Read the model definition and answer for the solid it produces. Units are mm, in the model's axes. Give positions to 0.01 mm unless a question says otherwise; leave off trailing zeros. Loops run counter-clockwise (first coordinate to the right, second up) from the corner with the lowest first, then second, coordinate; pieces in that order, holes last. Notation, with made-up numbers: (-12, 18.25) - (11, 18.25) arc R24 ccw to (11, 54.25) - close; hole circle Ø11 at (-31, 52.5). An arc over 180 degrees is marked (long way). Write item = value, one per line.
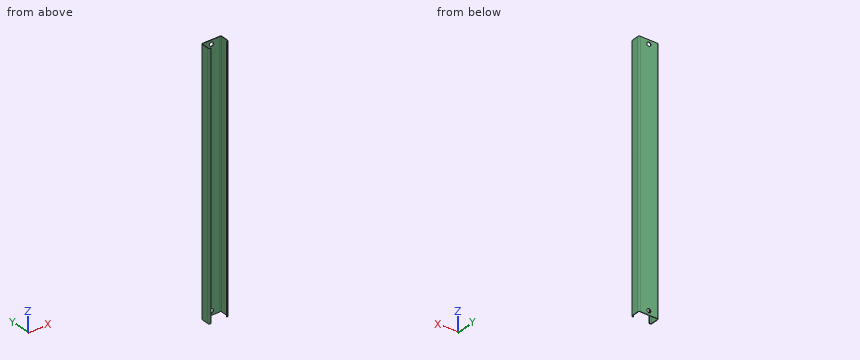
```python
from build123d import *

# Parameters (mm, degrees)
PAD001_DEPTH    = 572
SKETCH004_R     = 4.5
POCKET002_DEPTH = 5
SKETCH007_W     = 36
SKETCH007_H     = 572
POCKET004_DEPTH = 5


with BuildPart() as part:
    # Sketch003 → Pad001 (new body)
    with BuildSketch(Plane.XY):
        with BuildLine():
            Line((-19.5, 11), (19.5, 11))
            ThreePointArc((22, 8.5), (21.267767, 10.267767), (19.5, 11))
            Line((22, 8.5), (22, -8.5))
            ThreePointArc((19.5, -11), (21.267767, -10.267767), (22, -8.5))
            Line((19.5, -11), (-19.5, -11))
            ThreePointArc((-22, -8.5), (-21.267767, -10.267767), (-19.5, -11))
            Line((-22, -8.5), (-22, 8.5))
            ThreePointArc((-19.5, 11), (-21.267767, 10.267767), (-22, 8.5))
        make_face()
        with BuildLine():
            Line((-19.5, 10), (19.5, 10))
            ThreePointArc((21, 8.5), (20.56066, 9.56066), (19.5, 10))
            Line((21, 8.5), (21, -8.5))
            ThreePointArc((19.5, -10), (20.56066, -9.56066), (21, -8.5))
            Line((19.5, -10), (-19.5, -10))
            ThreePointArc((-21, -8.5), (-20.56066, -9.56066), (-19.5, -10))
            Line((-21, -8.5), (-21, 8.5))
            ThreePointArc((-19.5, 10), (-20.56066, 9.56066), (-21, 8.5))
        make_face(mode=Mode.SUBTRACT)
    extrude(amount=PAD001_DEPTH)

    # Sketch004 (on Face3 of Pad001) → Pocket002 (cut)
    with BuildSketch(Plane(origin=(0, 11, 0), x_dir=(-1, 0, 0), z_dir=(0, 1, 0))):
        with Locations((0, 9)):
            Circle(SKETCH004_R)
        with Locations((0, 563)):
            Circle(SKETCH004_R)
    extrude(amount=-POCKET002_DEPTH, mode=Mode.SUBTRACT)

    # Sketch007 (on Face6 of Pocket002) → Pocket004 (cut)
    with BuildSketch(Plane.XZ.offset(11)):
        with Locations((0, 286)):
            Rectangle(SKETCH007_W, SKETCH007_H)
    extrude(amount=-POCKET004_DEPTH, mode=Mode.SUBTRACT)


solid = part.part
```
1) A cutting plane is placed at A-A on y = 1.25. Determine the outline of the cut face in (x, z), then the cut area to 3 significant figures.
Output:
outline = (-22, 0) - (-21, 0) - (-21, 572) - (-22, 572) - close; (21, 0) - (22, 0) - (22, 572) - (21, 572) - close
area = 1,140 mm²
2) A cutting plane is placed at B-B on z = 94. Determine the outline of the cut face in (x, y).
Output:
outline = (-22, -8.5) arc R2.5 ccw to (-19.5, -11) - (-18, -11) - (-18, -10) - (-19.5, -10) arc R1.5 cw to (-21, -8.5) - (-21, 8.5) arc R1.5 cw to (-19.5, 10) - (19.5, 10) arc R1.5 cw to (21, 8.5) - (21, -8.5) arc R1.5 cw to (19.5, -10) - (18, -10) - (18, -11) - (19.5, -11) arc R2.5 ccw to (22, -8.5) - (22, 8.5) arc R2.5 ccw to (19.5, 11) - (-19.5, 11) arc R2.5 ccw to (-22, 8.5) - close
3) Each of these flat-tipped pins is pushed along its axis until it touches: P1, Ø10.5, axis at x = 0, z = 9, coming from the -Y side; P2, Ø0.5, axis at y = -10.5, z = 245, coming from the -X side. Where does it stop, or does it pass through?
Output:
P1 = 10
P2 = -21.29
4) Find the intervals of material crossed by probe 1 along Z at (x, y) = (0, 10.4); probe 2 along X at (y, z) = (9, 256.5); probe 3 along X at (y, z) = (-6.5, 176.5), in increasing order.
Output:
probe_1 = 0 to 4.5, 13.5 to 558.5, 567.5 to 572
probe_2 = -21.95 to -20.91, 20.91 to 21.95
probe_3 = -22 to -21, 21 to 22
